Model file for the job. Use its own axes, mm. A direction names the side the tool comes from. Give positions to 0.01 mm unless a question says otherwise; leave off trailing zeros. Order: outer loops, then holes, each group sorted by start corner. A loop starts at its lowest first (then second) coordinate and runs counter-clockwise, first axis right, second up. Notation, with made-up numbers: M -28.5,4 L -10.5,4 A29 cw -10.5,24 Z; hole C 25,42.5 d8. An arc over 180 degrees is marked long. Return JSON: item names as keys, results as strings. Group by question number.
1. Slice it at B-B on z = 26.5. Give the number of separate pieces and of enclosed holes in the cut face, then the cut area to 3 significant figures.
2. Two-plate mould, pull along Y, no slides. Class faces 3 (the face through (-13.986, 31.434, 14.297)), 4 (the face through (91.5, 16, 29)): released by +Y, released by -Y, zero draft, split by the parting line, or undercut.
3. Pin check, flat tips, straight feed: pin 1 (18.5 mm diameter, centred on x = 237, y = 17, fed in from -Z); pin 2 (1 mm diameter, centred on y = 52, z = 30, fed in from -X); pin 3 (7.5 mm diameter, centred on x = 37.5, y = 44, fed in from +Z); pin 4 (12 mm diameter, centred on x = 181.5, y = 16, fed in from +Z). Stop position of each tip, or through.
4. 3-axis set-ups, long thin cutter, end or side, ignore diameter. For faces 1 (the face through (45, 46, 2)), 2 (the face through (-7, 60, 7)): which of +Z, -Z, +X, -X, +Y, -Y reach the whole face in a straight line?
5. Slice it at A-A on x = 116.5. List the corners of the cut face in (y, z).
6. Slice it at C-C on y = 26.5. List the corners of the cut face in (x, z).
7. Wall check: probe 1 along Y at (x, z) = (30, 52); probe 2 along X at (y, z) = (35, 42.5); probe 3 along Y at (x, z) = (80, 8.5). Give the ranges that are in metal, low to high. Write a range as [from, to].
from build123d import *

# Parameters (mm, degrees)
PAD002_DEPTH                    = 62
SKETCH004_W                     = 87.5
SKETCH004_H                     = 28
POCKET001_DEPTH                 = 53
PAD_DEPTH                       = 87.5
SKETCH004_LINEARPATTERN_2_W     = 87.5
SKETCH004_LINEARPATTERN_2_H     = 28
POCKET001_LINEARPATTERN_2_DEPTH = 53
PAD_LINEARPATTERN_2_DEPTH       = 87.5
SKETCH004_LINEARPATTERN_3_W     = 87.5
SKETCH004_LINEARPATTERN_3_H     = 28
POCKET001_LINEARPATTERN_3_DEPTH = 53
PAD_LINEARPATTERN_3_DEPTH       = 87.5
SKETCH004_LINEARPATTERN_4_W     = 87.5
SKETCH004_LINEARPATTERN_4_H     = 28
POCKET001_LINEARPATTERN_4_DEPTH = 53
PAD_LINEARPATTERN_4_DEPTH       = 87.5
LINEARPATTERN001_COUNT          = 2
LINEARPATTERN001_PITCH          = 30
REVOLUTION_ANGLE                = -90


with BuildPart() as part:
    # Sketch006 → Pad002 (new body)
    with BuildSketch(Plane.XZ):
        Polygon((0, 55), (360, 55), (360, 0), (2, 0), (2, -7), (0, -7), align=None)
    extrude(amount=-PAD002_DEPTH)

    # Sketch004 (on DatumPlane) → Pocket001 (cut)
    with BuildSketch(Plane.XY.offset(55)):
        with Locations((45.75, 16)):
            Rectangle(SKETCH004_W, SKETCH004_H)
    pocket001 = extrude(amount=-POCKET001_DEPTH, mode=Mode.SUBTRACT)

    # Sketch (on DatumPlane) → Pad (join)
    with BuildSketch(Plane.YZ.offset(2)):
        with BuildLine():
            ThreePointArc((2, 11.333333), (4.73367, 4.73367), (11.333333, 2))
            Line((2, 2), (11.333333, 2))
            Line((2, 11.333333), (2, 2))
        make_face()
        with BuildLine():
            ThreePointArc((20.666667, 2), (27.26633, 4.73367), (30, 11.333333))
            Line((30, 2), (30, 11.333333))
            Line((20.666667, 2), (30, 2))
        make_face()
    pad = extrude(amount=PAD_DEPTH)

    # Sketch004 LinearPattern 2 → Pocket001 LinearPattern 2 (cut)
    with BuildSketch(Plane(origin=(89.5, 0, 55), x_dir=(1, 0, 0), z_dir=(0, 0, 1))):
        with Locations((45.75, 16)):
            Rectangle(SKETCH004_LINEARPATTERN_2_W, SKETCH004_LINEARPATTERN_2_H)
    pocket001_linearpattern_2 = extrude(amount=-POCKET001_LINEARPATTERN_2_DEPTH, mode=Mode.SUBTRACT)

    # Sketch LinearPattern 2 → Pad LinearPattern 2 (add)
    with BuildSketch(Plane.YZ.offset(91.5)):
        with BuildLine():
            ThreePointArc((2, 11.333333), (4.73367, 4.73367), (11.333333, 2))
            Line((2, 2), (11.333333, 2))
            Line((2, 11.333333), (2, 2))
        make_face()
        with BuildLine():
            ThreePointArc((20.666667, 2), (27.26633, 4.73367), (30, 11.333333))
            Line((30, 2), (30, 11.333333))
            Line((20.666667, 2), (30, 2))
        make_face()
    pad_linearpattern_2 = extrude(amount=PAD_LINEARPATTERN_2_DEPTH)

    # Sketch004 LinearPattern 3 → Pocket001 LinearPattern 3 (cut)
    with BuildSketch(Plane(origin=(179, 0, 55), x_dir=(1, 0, 0), z_dir=(0, 0, 1))):
        with Locations((45.75, 16)):
            Rectangle(SKETCH004_LINEARPATTERN_3_W, SKETCH004_LINEARPATTERN_3_H)
    pocket001_linearpattern_3 = extrude(amount=-POCKET001_LINEARPATTERN_3_DEPTH, mode=Mode.SUBTRACT)

    # Sketch LinearPattern 3 → Pad LinearPattern 3 (add)
    with BuildSketch(Plane.YZ.offset(181)):
        with BuildLine():
            ThreePointArc((2, 11.333333), (4.73367, 4.73367), (11.333333, 2))
            Line((2, 2), (11.333333, 2))
            Line((2, 11.333333), (2, 2))
        make_face()
        with BuildLine():
            ThreePointArc((20.666667, 2), (27.26633, 4.73367), (30, 11.333333))
            Line((30, 2), (30, 11.333333))
            Line((20.666667, 2), (30, 2))
        make_face()
    pad_linearpattern_3 = extrude(amount=PAD_LINEARPATTERN_3_DEPTH)

    # Sketch004 LinearPattern 4 → Pocket001 LinearPattern 4 (cut)
    with BuildSketch(Plane(origin=(268.5, 0, 55), x_dir=(1, 0, 0), z_dir=(0, 0, 1))):
        with Locations((45.75, 16)):
            Rectangle(SKETCH004_LINEARPATTERN_4_W, SKETCH004_LINEARPATTERN_4_H)
    pocket001_linearpattern_4 = extrude(amount=-POCKET001_LINEARPATTERN_4_DEPTH, mode=Mode.SUBTRACT)

    # Sketch LinearPattern 4 → Pad LinearPattern 4 (add)
    with BuildSketch(Plane.YZ.offset(270.5)):
        with BuildLine():
            ThreePointArc((2, 11.333333), (4.73367, 4.73367), (11.333333, 2))
            Line((2, 2), (11.333333, 2))
            Line((2, 11.333333), (2, 2))
        make_face()
        with BuildLine():
            ThreePointArc((20.666667, 2), (27.26633, 4.73367), (30, 11.333333))
            Line((30, 2), (30, 11.333333))
            Line((20.666667, 2), (30, 2))
        make_face()
    pad_linearpattern_4 = extrude(amount=PAD_LINEARPATTERN_4_DEPTH)

    # LinearPattern001: Pocket001, Pad, Pocket001 LinearPattern 2, Pad LinearPattern 2, Pocket001 LinearPattern 3, Pad LinearPattern 3, Pocket001 LinearPattern 4, Pad LinearPattern 4 ×2
    with Locations(*[(0, i * LINEARPATTERN001_PITCH, 0) for i in range(1, LINEARPATTERN001_COUNT)]):
        add(pocket001, mode=Mode.SUBTRACT)
        add(pad)
        add(pocket001_linearpattern_2, mode=Mode.SUBTRACT)
        add(pad_linearpattern_2)
        add(pocket001_linearpattern_3, mode=Mode.SUBTRACT)
        add(pad_linearpattern_3)
        add(pocket001_linearpattern_4, mode=Mode.SUBTRACT)
        add(pad_linearpattern_4)

    # Sketch007 → Revolution (revolve)
    with BuildSketch(Plane.YZ):
        Polygon((0, 0), (0, 20), (62, 20), (62, 0), (60, 0), (60, 18), (2, 18), (2, 0), align=None)
    revolve(axis=Axis((0, 0, 0), (0, 1, 0)), revolution_arc=REVOLUTION_ANGLE)


solid = part.part
Result:
{
 "1": {"separate pieces": "1", "enclosed holes": "8", "area": "2,720 mm2"},
 "2": {"face 3": "zero draft", "face 4": "undercut"},
 "3": {"pin 1": "stops at z = 0", "pin 2": "stops at x = 0", "pin 3": "stops at z = 2.06", "pin 4": "stops at z = 55"},
 "4": {"face 1": "+Z", "face 2": "-Z"},
 "5": {"outline": "M 0,0 L 62,0 L 62,55 L 60,55 L 60,11.33 A9.33 cw 50.67,2 L 41.33,2 A9.33 cw 32,11.33 L 32,55 L 30,55 L 30,11.33 A9.33 cw 20.67,2 L 11.33,2 A9.33 cw 2,11.33 L 2,55 L 0,55 Z"},
 "6": {"outline": "M -20,0 L -18,0 A18 cw 0,18 L 0,-7 L 2,-7 L 2,0 L 360,0 L 360,55 L 358,55 L 358,4.05 L 270.5,4.05 L 270.5,55 L 268.5,55 L 268.5,4.05 L 181,4.05 L 181,55 L 179,55 L 179,4.05 L 91.5,4.05 L 91.5,55 L 89.5,55 L 89.5,4.05 L 2,4.05 L 2,55 L 0,55 L 0,20 A20 ccw Z"},
 "7": {"probe 1": "y = [0, 2], [30, 32], [60, 62]", "probe 2": "x = [0, 2], [89.5, 91.5], [179, 181], [268.5, 270.5], [358, 360]", "probe 3": "y = [0, 2.44], [29.56, 32.44], [59.56, 62]"}
}
